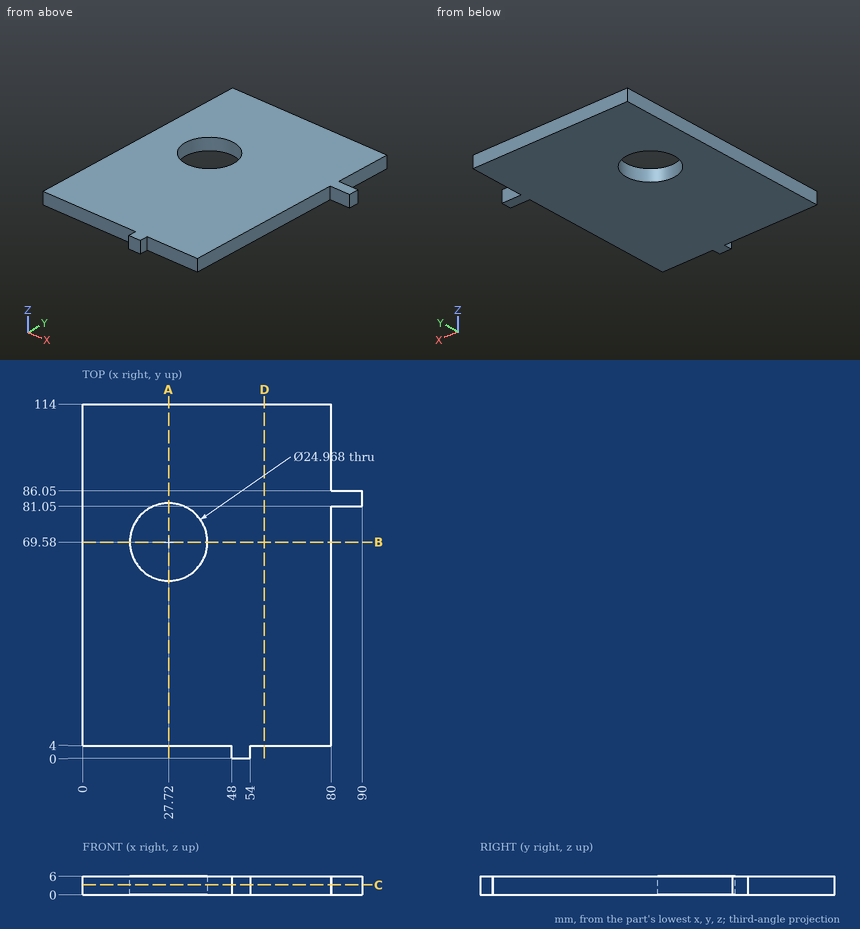
For this review, use the dimensioned drawing (mm, ordinates from the lowest corner) and the shaded views. Coordinates: 2 decimals unless noted, no trailing zeros. Loops run counter-clockwise (first coordinate to the right, second up) from the corner with the lowest first, then second, coordinate; pieces in that order, holes last. Notation, with made-up numbers: (44.5, 75) -> (62.5, 75) arc R8 ccw to (62.5, 82) -> close; hole circle Ø11 at (-29.75, 19.5). An arc over 180 degrees is marked (long way). Use a Markdown table: item, result. Add a question column.
1. To check wall thickness, follow line 1 (Y direction, x = 27.72, z = 3.55); line 2 (Y direction, x = 11.5, z = 3); line 3 (X direction, y = 21.5, z = 5.5). State the ranges of each line that lie inside material, in increasing order.
2. Add section A-A on x = 27.72. Write out the cut boundary in (y, z), plus the area to 3 significant figures.
3. Add section B-B on y = 69.58. Write out the cut boundary in (x, z).
4. Add section D-D on x = 58.5. Write out the cut boundary in (y, z).
5. Clearance check with flat-ended pins moving along their axes: pin 1 Ø1.8 at (x, z) = (82.5, 2.5) entering from -Y; pin 2 Ø1.2 at (y, z) = (2.5, 4) entering from +X; pin 3 Ø1.8 at (x, z) = (69, 2.5) entering from -Y; pin 4 Ø5 at (x, y) = (32.5, 76) entering from -Z. State where each tip first meets the part, or that it passes through.
6. Add section C-C on z = 3.25. Write out the cut boundary in (x, y), plus the area to 3 significant figures.
Returned:
| question | item | result |
|---|---|---|
| 1 | line 1 | y = 4 to 57.1, 82.06 to 114 |
| 1 | line 2 | y = 4 to 114 |
| 1 | line 3 | x = 0 to 80 |
| 2 | outline | (4, 0) -> (57.1, 0) -> (57.1, 6) -> (4, 6) -> close; (82.06, 0) -> (114, 0) -> (114, 6) -> (82.06, 6) -> close |
| 2 | area | 510 mm² |
| 3 | outline | (0, 0) -> (15.24, 0) -> (15.24, 6) -> (0, 6) -> close; (40.2, 0) -> (80, 0) -> (80, 6) -> (40.2, 6) -> close |
| 4 | outline | (4, 0) -> (114, 0) -> (114, 6) -> (4, 6) -> close |
| 5 | pin 1 | stops at y = 81.05 |
| 5 | pin 2 | stops at x = 54 |
| 5 | pin 3 | stops at y = 4 |
| 5 | pin 4 | passes through |
| 6 | outline | (0, 4) -> (48, 4) -> (48, 0) -> (54, 0) -> (54, 4) -> (80, 4) -> (80, 81.05) -> (90, 81.05) -> (90, 86.05) -> (80, 86.05) -> (80, 114) -> (0, 114) -> close; hole circle Ø24.97 at (27.72, 69.58) |
| 6 | area | 8,380 mm² |
